```python
from build123d import *

# Parameters (mm, degrees)
EXTRUDE_THIN1_DEPTH = 841.375
FILLET1_R           = 1.27


with BuildPart() as part:
    # Sketch1 → Extrude-Thin1 (new body)
    with BuildSketch(Plane.XY):
        with BuildLine():
            Line((0, 0), (-21.43125, 0))
            Line((-21.43125, 0), (-21.43125, 30.62560856))
            ThreePointArc((-21.43125, 30.62560856), (-25.982145735, 45.62307319), (-38.1, 55.5625))
            Line((-38.1, 55.5625), (-38.1, 84.1375))
            Line((-38.1, 84.1375), (0, 84.1375))
            Line((0, 84.1375), (0, 82.8675))
            Line((0, 82.8675), (-36.83, 82.8675))
            Line((-36.83, 82.8675), (-36.83, 56.397437748))
            ThreePointArc((-36.83, 56.397437748), (-24.691598787, 45.971898065), (-20.16125, 30.62560856))
            Line((-20.16125, 30.62560856), (-20.16125, 1.27))
            Line((-20.16125, 1.27), (0, 1.27))
            Line((0, 1.27), (0, 0))
        make_face()
    extrude(amount=-EXTRUDE_THIN1_DEPTH)

    # Fillet1
    fillet1_edges = [part.edges().sort_by_distance(p)[0] for p in [
        (-21.43125, 0, -420.6875),
        (-38.1, 55.5625, -420.6875),
        (-38.1, 84.1375, -420.6875),
    ]]
    fillet(fillet1_edges, radius=FILLET1_R)


solid = part.part
```
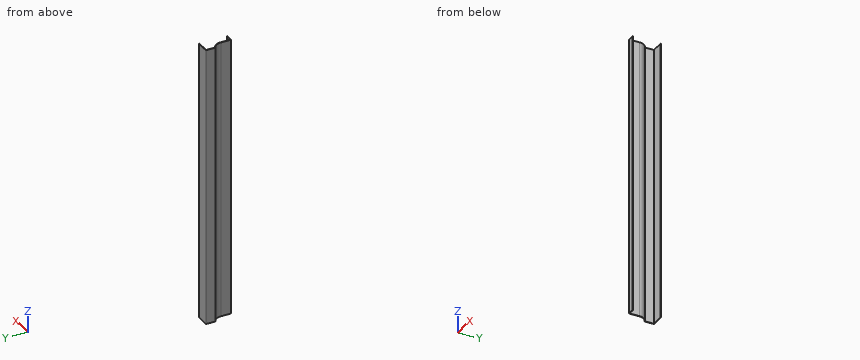
Can you work these out from the model? Positions are in its coordinate system, mm. Round coordinates to 2 decimals unless told otherwise and drop trailing zeros. Loops run counter-clockwise (first coordinate to the right, second up) from the corner with the lowest first, then second, coordinate; pieces in that order, holes last. Notation, with made-up numbers: (-13.5, 23.5) -> (15.5, 23.5) arc R15 ccw to (15.5, 37.5) -> close; hole circle Ø4 at (54, 2). An arc over 180 degrees is marked (long way). Answer in a Markdown table with one row per item.
Item 1: Suppose I cut it at C-C, the plane y = 23. List the corners of the cut face in (x, z) for me (3 decimals).
Answer block:
| item | result |
|---|---|
| outline | (-21.431, -841.375) -> (-20.161, -841.375) -> (-20.161, 0) -> (-21.431, 0) -> close |
Item 2: Will these pins go through, and if not, where does the flat tip stop? P1, Ø3, axis at y = 33, z = -293, coming from the +X side; P2, Ø1.5, axis at y = 67.5, z = -515.5, coming from the +X side; P3, Ø21, axis at y = 66.5, z = -418, coming from the +X side; P4, Ø8, axis at x = -17.5, y = 20, coming from the +Z side.
Answer block:
| item | result |
|---|---|
| P1 | x = -20.17 |
| P2 | x = -36.83 |
| P3 | x = -35.98 |
| P4 | z = 0 |
Item 3: Suppose I cut it at A-A, the plane x = -8.5. List the corners of the cut face in (y, z) for me (1 decimal).
Answer block:
| item | result |
|---|---|
| outline | (0, -841.4) -> (1.3, -841.4) -> (1.3, 0) -> (0, 0) -> close; (82.9, -841.4) -> (84.1, -841.4) -> (84.1, 0) -> (82.9, 0) -> close |
Item 4: Suppose I cut it at B-B, the plane z = -403. List the corners of the cut face in (x, y) for me (1 decimal).
Answer block:
| item | result |
|---|---|
| outline | (-38.1, 56.4) arc R1.3 ccw to (-37.4, 55.2) arc R27 cw to (-21.4, 30.6) -> (-21.4, 1.3) arc R1.3 ccw to (-20.2, 0) -> (0, 0) -> (0, 1.3) -> (-20.2, 1.3) -> (-20.2, 30.6) arc R28.3 ccw to (-36.8, 56.4) -> (-36.8, 82.9) -> (0, 82.9) -> (0, 84.1) -> (-36.8, 84.1) arc R1.3 ccw to (-38.1, 82.9) -> close |
Item 5: If I drill on probe 1 along Y at (x, z) = (-19.5, -319); probe 2 along X at (y, z) = (28, -636); probe 3 along X at (y, z) = (78.5, -642.5), over which ranges is the centre line in solid material (lowest first)?
Answer block:
| item | result |
|---|---|
| probe 1 | 0 to 1.27, 82.87 to 84.14 |
| probe 2 | -21.43 to -20.16 |
| probe 3 | -38.1 to -36.83 |
